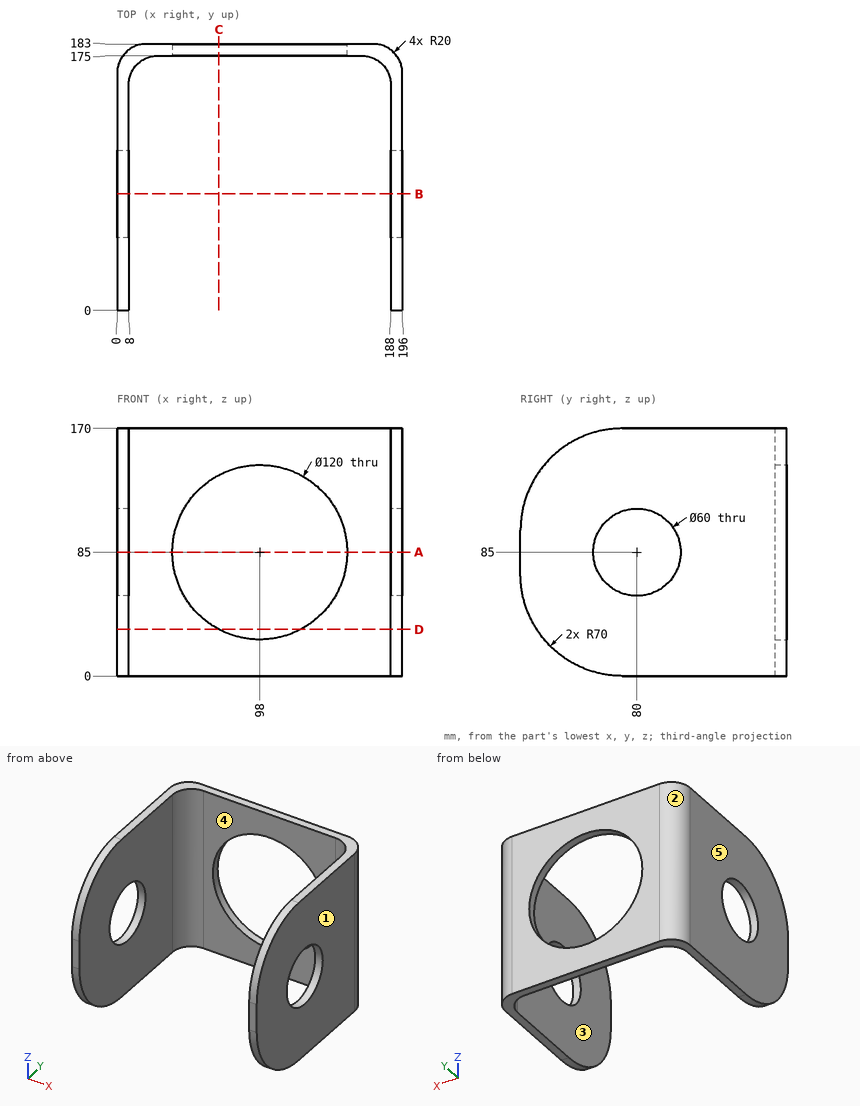
Geometry check sheet. Reference: drawing and pictorial views, mm from the part's lowest x, y, z. A direction names the side the tool comes from. Coordinates: 2 decimals unless noted, no trailing zeros. Order: outer loops, then holes, each group sorted by start corner. A loop starts at its lowest first (then second) coordinate and runs counter-clockwise, first axis right, second up. Notation, with made-up numbers: (39.5, -27.75) - (49.5, -27.75) arc R30 cw to (49.5, 2.25) - close; hole circle Ø9 at (29, -22). An arc over 180 degrees is marked (long way). Answer in a Markdown table with one row per item. Add a question column.
1) Cross-section at B-B, the plane y = 80. Record the cut outline in (x, z).
2) Cross-section at A-A, the plane z = 85. Record the cut outline in (x, y), then the cut area to 3 significant figures.
3) Release check for a two-part mould opening along X. For the marked faces 1, 2 and 3 record: +X half, -X half, draft (parallel to the pull), parting line (faces both ways), or undercut.
4) Set-up check for the marked faces 4 and 5: record each of +Z, -Z, +X, -X, +Y, -Y from which the full face is reachable in a straight line by a thin tool's end or side.
5) Cross-section at C-C, the plane x = 70. Record the cut outline in (y, z), then the cut area to 3 significant figures.
6) Cross-section at D-D, the plane z = 32. Record the cut outline in (x, y), then the cut area to 3 significant figures.
7) Material ranges on line 1 along X through (y, z) = (72, 161.5); line 2 along Z through (x, y) = (98, 177.75); line 3 along Z through (x, y) = (193.75, 80), recorded low to high. Write a range as [from, to].
Check result:
| question | item | result |
|---|---|---|
| 1 | outline | (0, 0) - (8, 0) - (8, 55) - (0, 55) - close; (0, 115) - (8, 115) - (8, 170) - (0, 170) - close; (188, 0) - (196, 0) - (196, 55) - (188, 55) - close; (188, 115) - (196, 115) - (196, 170) - (188, 170) - close |
| 2 | outline | (0, 0) - (8, 0) - (8, 50) - (0, 50) - close; (0, 110) - (8, 110) - (8, 155) arc R20 cw to (28, 175) - (38, 175) - (38, 183) - (20, 183) arc R20 ccw to (0, 163) - close; (158, 175) - (168, 175) arc R20 cw to (188, 155) - (188, 110) - (196, 110) - (196, 163) arc R20 ccw to (176, 183) - (158, 183) - close; (188, 0) - (196, 0) - (196, 50) - (188, 50) - close |
| 2 | area | 2,450 mm² |
| 3 | face 1 | +X half |
| 3 | face 2 | -X half |
| 3 | face 3 | undercut |
| 4 | face 4 | +Z, -Z, -Y |
| 4 | face 5 | +Z, -Z, -X, +Y, -Y |
| 5 | outline | (175, 0) - (183, 0) - (183, 31.93) - (175, 31.93) - close; (175, 138.07) - (183, 138.07) - (183, 170) - (175, 170) - close |
| 5 | area | 511 mm² |
| 6 | outline | (0, 11.21) - (8, 11.21) - (8, 155) arc R20 cw to (28, 175) - (69.88, 175) - (69.88, 183) - (20, 183) arc R20 ccw to (0, 163) - close; (126.12, 175) - (168, 175) arc R20 cw to (188, 155) - (188, 11.21) - (196, 11.21) - (196, 163) arc R20 ccw to (176, 183) - (126.12, 183) - close |
| 6 | area | 3,740 mm² |
| 7 | line 1 | x = [0, 8], [188, 196] |
| 7 | line 2 | z = [0, 25], [145, 170] |
| 7 | line 3 | z = [0, 55], [115, 170] |
